For this review, take the finished solid that the model builds, in its own axes (mm). A direction names the side the tool comes from. Give positions to 0.01 mm unless a question says otherwise; leave off trailing zeros. Order: outer loops, then holes, each group sorted by start corner. A loop starts at its lowest first (then second) coordinate and runs counter-clockwise, first axis right, second up. Notation, with made-up numbers: (-13.5, 37) -> (-2.5, 37) arc R14 cw to (-2.5, 53) -> close; hole circle Ø1 at (31, 17.25). An arc over 180 degrees is marked (long way). Use CSV: the item, a comma, the result in double quotes. Start each with the question number.
Autodesk Inventor part; units mm, degrees
ref_plane "YZ Plane" through (0, 0, 0) normal (1, 0, 0) x (0, 1, 0)
ref_plane "XZ Plane" through (0, 0, 0) normal (0, 1, 0) x (-1, 0, 0)
ref_plane "XY Plane" through (0, 0, 0) normal (0, 0, 1) x (1, 0, 0)
sketch "Skizze1" plane through (0, 0, 0) normal (0, 1, 0) x (-1, 0, 0)
  line L0 (22.5, 22.5) -> (-22.5, 22.5)
  line L1 (-22.5, 22.5) -> (-22.5, -22.5)
  line L2 (-22.5, -22.5) -> (22.5, -22.5)
  line L3 (22.5, -22.5) -> (22.5, 22.5)
  line L4 (17.5, 17.5) -> (-17.5, 17.5) construction
  line L5 (-17.5, 17.5) -> (-17.5, -17.5) construction
  line L6 (-17.5, -17.5) -> (17.5, -17.5) construction
  line L7 (17.5, -17.5) -> (17.5, 17.5) construction
  circle A0 centre (17.5, 17.5) radius 1.5
  circle A1 centre (17.5, -17.5) radius 1.5
  circle A2 centre (-17.5, 17.5) radius 1.5
  circle A3 centre (-17.5, -17.5) radius 1.5
  point P0 (0, 0)
  point P1 (0, 22.5)
  point P2 (22.5, 0)
  dimension "d0" = 45
  dimension "d1" = 5
  dimension "d2" = 35
  dimension "d3" = 3
extrude "Extrusion1" add sketch "Skizze1" along normal blind 3
sketch "Skizze2" plane through (0, 3, 0) normal (0, 1, 0) x (1, 0, 0)
  line L0 (-15, -15) -> (15, -15)
  line L1 (15, -15) -> (15, 15)
  line L2 (15, 15) -> (-15, 15)
  line L3 (-15, 15) -> (-15, -15)
  point P0 (0, 0)
  point P1 (0, -15)
  point P2 (-15, 0)
  dimension "d7" = 30
extrude "Extrusion2" add sketch "Skizze2" along normal blind 30
sketch "Skizze3" plane through (15, 3, 15) normal (1, 0, 0) x (0, 0, -1)
  circle A0 centre (15, 22.5) radius 15
  line L0 (-7.5, 0) -> (37.5, 0) construction
  line L1 (-7.5, -3) -> (37.5, -3)
  point P0 (15, -3)
  point P1 (15, -3)
  point P2 (15, 0)
  point P3 (15, 7.5)
  point P4 (15, 0)
  point P5 (15, -3)
  dimension "d10" = 30
  dimension "d18" = 7.5
extrude "Extrusion3" cut sketch "Skizze3" against normal through all
sketch "Skizze4" plane through (15, 3, -15) normal (1, 0, 0) x (0, 0, -1)
  line L0 (0, 30) -> (-30, 30)
  line L1 (-30, 30) -> (-30, 15)
  line L2 (-30, 15) -> (0, 15)
  line L3 (0, 15) -> (0, 30)
  arc A0 (-27.9904, 30) -> (-2.0096, 30) centre (-15, 22.5) ccw construction
  point P0 (-15, -3)
  point P1 (-15, 0)
  dimension "d24" = 15
extrude "Extrusion4" cut sketch "Skizze4" against normal through all
sketch "Skizze5" plane through (15, 3, -15) normal (0, 0, -1) x (-1, 0, 0)
  line L0 (27.5, 5) -> (2.5, 5)
  line L1 (2.5, 5) -> (2.5, 2)
  line L2 (2.5, 2) -> (27.5, 2)
  line L3 (27.5, 2) -> (27.5, 5)
  line L4 (-7.5, 0) -> (37.5, 0) construction
  point P0 (15, -3)
  point P1 (15, 2)
  dimension "d19" = 25
  dimension "d20" = 3
  dimension "d21" = 2
extrude "Extrusion5" cut sketch "Skizze5" against normal through all
properties part number "fastening-clip" material "PC/ABS-Kunststoff"
1. To check wall thickness, follow L1, parallel to Z at x = 17.5, y = 0.7; L2, parallel to Y at x = 6, z = -14; L3, parallel to X at y = 1.25, z = 17. State the ranges of each line that lie inside material, in increasing order. Write a range as [from, to].
2. Consider section D-D (x = 17.5). State the section outline as (y, z) points.
3. Clearance check with flat-ended pins moving along their axes: P1, Ø7.5, axis at x = 2.5, z = -3, coming from the +Y side; P2, Ø1.5, axis at y = 7, z = -4.5, coming from the +X side; P3, Ø3.5, axis at y = 7, z = 4.5, coming from the -X side; P4, Ø3, axis at x = 18, y = 15.5, coming from the -Z side. State where each tip first meets the part, or that it passes through.
4. For faces 1 (the face through (18.61, 1.48, -18.51)), 2 (the face through (15, 9, 0)), 3 (the face through (0, 8, 0)), list the 3-axis set-ups (+Z, -Z, +X, -X, +Y, -Y) from which the entire face can be reached by the end or side of a thin tool; tool diameter is ignored.
5. Consider section B-B (z = -17.5). State the section outline as (x, y) points.
6. Draft analysis for pull direction Z (two halves, no side actions). For faces 4 (the face through (18.61, 1.48, 16.49)), 5 (the face through (-15, 9, 0)), 6 (the face through (0, 12, -15)), state which applies: +Z half, -Z half, draft (parallel to the pull), parting line (faces both ways), or undercut.
7. Consider section A-A (y = 13.5). State the section outline as (x, z) points, plus the area to 3 significant figures.
8. Consider section C-C (x = -3). State the section outline as (y, z) points.
Answer list:
1,L1,"[-22.5, -19], [-16, 16], [19, 22.5]"
1,L2,"[0, 5], [8, 18]"
1,L3,"[-22.5, -18.91], [-16.09, 16.09], [18.91, 22.5]"
2,outline,"(0, -22.5) -> (3, -22.5) -> (3, -19) -> (0, -19) -> close; (0, -16) -> (3, -16) -> (3, 16) -> (0, 16) -> close; (0, 19) -> (3, 19) -> (3, 22.5) -> (0, 22.5) -> close"
3,P1,"y = 12.1"
3,P2,"x = 15"
3,P3,"x = -15"
3,P4,"through"
4,face 1,"+Y, -Y"
4,face 2,"+Z, -Z, +X, +Y"
4,face 3,"+Z, -Z"
5,outline,"(-22.5, 0) -> (-19, 0) -> (-19, 3) -> (-22.5, 3) -> close; (-16, 0) -> (16, 0) -> (16, 3) -> (-16, 3) -> close; (19, 0) -> (22.5, 0) -> (22.5, 3) -> (19, 3) -> close"
6,face 4,"undercut"
6,face 5,"draft"
6,face 6,"-Z half"
7,outline,"(-15, -15) -> (15, -15) -> (15, -9) -> (-15, -9) -> close; (-15, 9) -> (15, 9) -> (15, 15) -> (-15, 15) -> close"
7,area,"360 mm2"
8,outline,"(0, -22.5) -> (3, -22.5) -> (3, -15) -> (5, -15) -> (5, 15) -> (3, 15) -> (3, 22.5) -> (0, 22.5) -> close; (8, -15) -> (18, -15) -> (18, -12.99) arc R15 cw to (18, 12.99) -> (18, 15) -> (8, 15) -> close"
